Build history of the part. All positions in model axes, mm. A direction names the side the tool comes from. Round coordinates to 2 decimals unless told otherwise and drop trailing zeros. Write each loop counter-clockwise with the first axis right and the second up, starting at its lowest first coordinate (ties: lowest second). Pieces come first, ordered by that corner, then holes. Notation, with made-up numbers: M -29.5,-21.5 L -22.5,-21.5 A20 ccw -22.5,14.5 Z; hole C 21.25,-38 d4. An arc over 180 degrees is marked long. Write item = value, one per line. Start each with the question number.
Q1. Probe L1, parallel to Y at x = 20.5, z = -3; L2, parallel to X at y = 77, z = -12.75; L3, parallel to Z at x = 50, y = 60.5. List the from-to ranges inside material, lowest first.
Q2. Band-saw the part on B-B on y = 143. Write the cut outline in (x, z), plus the area to 3 significant figures.
Q3. Pull direction Y, two halves, no side cores. Call faces 1 (the cylindrical face through (10.254, 56.769, -8.052)), 2 (the cylindrical face through (12.119, 170.523, -7.805)), 3 (the flat face through (15, 123, -18.332)): released by +Y, released by -Y, zero draft, split by the parting line, or undercut.
Q4. Tool access for faces 4 (the flat face through (32.979, 144, -17)), 5 (the cylindrical face through (33.68, 55.3, -5.42)), 6 (the flat face through (16.116, 152, -17)): list every direction of +Z, -Z, +X, -X, +Y, -Y with a clear straight run to the whole face (end or side of a thin tool).
Q5. Drop flat-ended pins along their axis: P1, Ø5, axis at x = 36.9, z = -5, coming from the -Y side; P2, Ø1.8, axis at x = 50.5, z = -16.5, coming from the -Y side; P3, Ø1.6, axis at x = 43.5, z = -17.5, coming from the +Y side; P4, Ø13, axis at x = 40, y = 161, coming from the +Z side. Give the stop position or say it passes through.
Q6. Band-saw the part on C-C on z = -5. State how many separate pieces and enclosed holes the cut face has, plus the area to 3 significant figures.
Q7. Band-saw the part on A-A on y = 161.5. Write the cut outline in (x, z).
Q8. Band-saw the part on D-D on y = 117. Write the cut outline in (x, z), plus the area to 3 significant figures.
```python
from build123d import *

# Parameters (mm, degrees)
BOSS_EXTRUDE1_DEPTH = 18.332422662
SHELL2_T            = -2.5
SKETCH2_W           = 26.4
SKETCH2_H           = 19.1
SKETCH2_W_2         = 13
SKETCH2_H_2         = 13
SKETCH2_W_3         = 38.578
SKETCH2_H_3         = 76.372933558
CUT_EXTRUDE1_DEPTH  = 4
FILLET1_R           = 2
FILLET2_R           = 1.2
FILLET4_R           = 1
CUT_EXTRUDE2_REACH  = 186.618
SKETCH3_W           = 10.732422662
SKETCH3_H           = 15
FILLET5_R           = 1
SKETCH6_W           = 26.474005188
SKETCH6_H           = 27.4
CUT_EXTRUDE5_DEPTH  = 2.2
SKETCH7_R           = 3.25
CUT_EXTRUDE6_DEPTH  = 1.6
SKETCH8_R           = 3.25
CUT_EXTRUDE7_DEPTH  = 1.6
SKETCH9_R           = 1.5
CUT_EXTRUDE8_DEPTH  = 5
SKETCH10_R          = 1.5
CUT_EXTRUDE9_DEPTH  = 5


with BuildPart() as part:
    # Sketch1 → Boss-Extrude1 (new body)
    with BuildSketch(Plane.XY):
        with BuildLine():
            Line((15.615664433, 54.513874967), (58.193664433, 54.513874967))
            ThreePointArc((58.193664433, 54.513874967), (63.496965292, 56.710574108), (65.693664433, 62.013874967))
            Line((65.693664433, 62.013874967), (65.693664433, 166.948874967))
            ThreePointArc((65.693664433, 166.948874967), (63.496965292, 172.252175826), (58.193664433, 174.448874967))
            Line((58.193664433, 174.448874967), (15.615664433, 174.448874967))
            ThreePointArc((15.615664433, 174.448874967), (10.312363574, 172.252175826), (8.115664433, 166.948874967))
            Line((8.115664433, 166.948874967), (8.115664433, 62.013874967))
            ThreePointArc((8.115664433, 62.013874967), (10.312363574, 56.710574108), (15.615664433, 54.513874967))
        make_face()
    extrude(amount=-BOSS_EXTRUDE1_DEPTH)

    # Shell2
    shell2_openings = [part.faces().sort_by_distance(p)[0] for p in [
        (36.904664433, 114.481374967, 0),
    ]]
    offset(amount=SHELL2_T, openings=shell2_openings, kind=Kind.INTERSECTION)

    # Sketch2 → Cut-Extrude1 (cut)
    with BuildSketch(Plane(origin=(0, 0, -18.332422662), x_dir=(-1, 0, 0), z_dir=(0, 0, -1))):
        with Locations((-45.679251594, 154.936808525)):
            Rectangle(SKETCH2_W, SKETCH2_H)
        with Locations((-22.615664433, 152.448874967)):
            Rectangle(SKETCH2_W_2, SKETCH2_H_2)
        with Locations((-36.904664433, 102.200341746)):
            Rectangle(SKETCH2_W_3, SKETCH2_H_3)
    extrude(amount=-CUT_EXTRUDE1_DEPTH, mode=Mode.SUBTRACT)

    # Fillet1
    fillet1_edges = [part.edges().sort_by_distance(p)[0] for p in [
        (63.496965292, 56.710574108, -18.332422662),
        (65.693664433, 114.481374967, -18.332422662),
        (63.496965292, 172.252175826, -18.332422662),
        (36.904664433, 174.448874967, -18.332422662),
        (10.312363574, 172.252175826, -18.332422662),
        (8.115664433, 114.481374967, -18.332422662),
        (10.312363574, 56.710574108, -18.332422662),
        (36.904664433, 54.513874967, -18.332422662),
    ]]
    fillet(fillet1_edges, radius=FILLET1_R)

    # Fillet2
    fillet2_edges = [part.edges().sort_by_distance(p)[0] for p in [
        (36.904664433, 64.013874967, -15.832422662),
        (17.615664433, 102.200341746, -15.832422662),
        (36.904664433, 140.386808525, -15.832422662),
        (56.193664433, 102.200341746, -15.832422662),
        (56.193664433, 102.200341746, -18.332422662),
        (36.904664433, 64.013874967, -18.332422662),
        (17.615664433, 102.200341746, -18.332422662),
        (36.904664433, 140.386808525, -18.332422662),
    ]]
    fillet(fillet2_edges, radius=FILLET2_R)

    # Fillet4
    fillet4_edges = [part.edges().sort_by_distance(p)[0] for p in [
        (45.679251594, 164.486808525, -15.832422662),
        (45.679251594, 145.386808525, -15.832422662),
        (32.479251594, 154.936808525, -18.332422662),
        (45.679251594, 164.486808525, -18.332422662),
        (58.879251594, 154.936808525, -18.332422662),
    ]]
    fillet(fillet4_edges, radius=FILLET4_R)

    # Sketch3 → Cut-Extrude2 (cut, up to next)
    with BuildSketch(Plane(origin=(65.693664433, 0, 0), x_dir=(0, 0, -1), z_dir=(1, 0, 0)), mode=Mode.PRIVATE) as cut_extrude2_sk1:
        with Locations((5.366211331, 156.448874967)):
            Rectangle(SKETCH3_W, SKETCH3_H)
    cut_extrude2_tool1 = extrude(cut_extrude2_sk1.sketch, amount=-CUT_EXTRUDE2_REACH, mode=Mode.PRIVATE) & part.part
    add(cut_extrude2_tool1.solids().sort_by_distance((65.693664, 156.448875, -5.366211))[0], mode=Mode.SUBTRACT)

    # Fillet5
    fillet5_edges = [part.edges().sort_by_distance(p)[0] for p in [
        (65.693664433, 148.948874967, -5.366211331),
        (65.693664433, 156.448874967, -10.732422662),
        (65.693664433, 163.948874967, -5.366211331),
    ]]
    fillet(fillet5_edges, radius=FILLET5_R)

    # Sketch6 → Cut-Extrude5 (cut)
    with BuildSketch(Plane.XY.offset(-15.832422662)):
        with Locations((46.216254188, 155.386808525)):
            Rectangle(SKETCH6_W, SKETCH6_H)
    extrude(amount=-CUT_EXTRUDE5_DEPTH, mode=Mode.SUBTRACT)

    # Sketch7 → Cut-Extrude6 (cut)
    with BuildSketch(Plane(origin=(0, 174.448874967, 0), x_dir=(1, 0, 0), z_dir=(0, 1, 0))):
        with Locations(Location((36.904664433, 5, 0), (0, 0, 270))):
            Circle(SKETCH7_R)
    extrude(amount=-CUT_EXTRUDE6_DEPTH, mode=Mode.SUBTRACT)

    # Sketch8 → Cut-Extrude7 (cut)
    with BuildSketch(Plane.XZ.offset(-54.513874967)):
        with Locations(Location((36.904664433, -5, 0), (0, 0, 90))):
            Circle(SKETCH8_R)
    extrude(amount=-CUT_EXTRUDE7_DEPTH, mode=Mode.SUBTRACT)

    # Sketch9 → Cut-Extrude8 (cut)
    with BuildSketch(Plane.XZ.offset(-56.113874967)):
        with Locations(Location((36.904664433, -5, 0), (0, 0, 270))):
            Circle(SKETCH9_R)
    extrude(amount=-CUT_EXTRUDE8_DEPTH, mode=Mode.SUBTRACT)

    # Sketch10 → Cut-Extrude9 (cut)
    with BuildSketch(Plane(origin=(0, 172.848874967, 0), x_dir=(1, 0, 0), z_dir=(0, 1, 0))):
        with Locations(Location((36.904664433, 5, 0), (0, 0, 90))):
            Circle(SKETCH10_R)
    extrude(amount=-CUT_EXTRUDE9_DEPTH, mode=Mode.SUBTRACT)


solid = part.part
```
Conclusion:
q1.L1 = 54.51 to 57.01, 171.95 to 174.45
q1.L2 = 8.12 to 10.62, 63.19 to 65.69
q1.L3 = -18.33 to -15.83
q2.outline = M 8.12,-16.33 A2 ccw 10.12,-18.33 L 63.69,-18.33 A2 ccw 65.69,-16.33 L 65.69,0 L 63.19,0 L 63.19,-15.83 L 59.45,-15.83 L 59.45,-18.03 L 32.98,-18.03 L 32.98,-15.83 L 10.62,-15.83 L 10.62,0 L 8.12,0 Z
q2.area = 163 mm^2
q3.face_1 = released by -Y
q3.face_2 = undercut
q3.face_3 = zero draft
q4.face_4 = +Z
q4.face_5 = -Y
q4.face_6 = +Z, -Z
q5.P1 = 56.11
q5.P2 = 54.51
q5.P3 = 174.41
q5.P4 = -18.03
q6.separate_pieces = 3
q6.enclosed_holes = 0
q6.area = 772 mm^2
q7.outline = M 8.12,-16.33 A2 ccw 10.12,-18.33 L 31.48,-18.33 A1 ccw 32.48,-17.33 L 32.48,-15.83 L 10.62,-15.83 L 10.62,0 L 8.12,0 Z; M 59.17,-18.03 A1 ccw 59.88,-18.33 L 63.69,-18.33 A2 ccw 65.69,-16.33 L 65.69,-11.73 A1 ccw 64.69,-10.73 L 63.19,-10.73 L 63.19,-15.83 L 59.45,-15.83 L 59.45,-18.03 Z
q8.outline = M 8.12,-16.33 A2 ccw 10.12,-18.33 L 16.42,-18.33 A1.2 ccw 17.62,-17.13 L 17.62,-17.03 A1.2 ccw 16.42,-15.83 L 10.62,-15.83 L 10.62,0 L 8.12,0 Z; M 56.19,-17.13 A1.2 ccw 57.39,-18.33 L 63.69,-18.33 A2 ccw 65.69,-16.33 L 65.69,0 L 63.19,0 L 63.19,-15.83 L 57.39,-15.83 A1.2 ccw 56.19,-17.03 Z
q8.area = 124 mm^2
